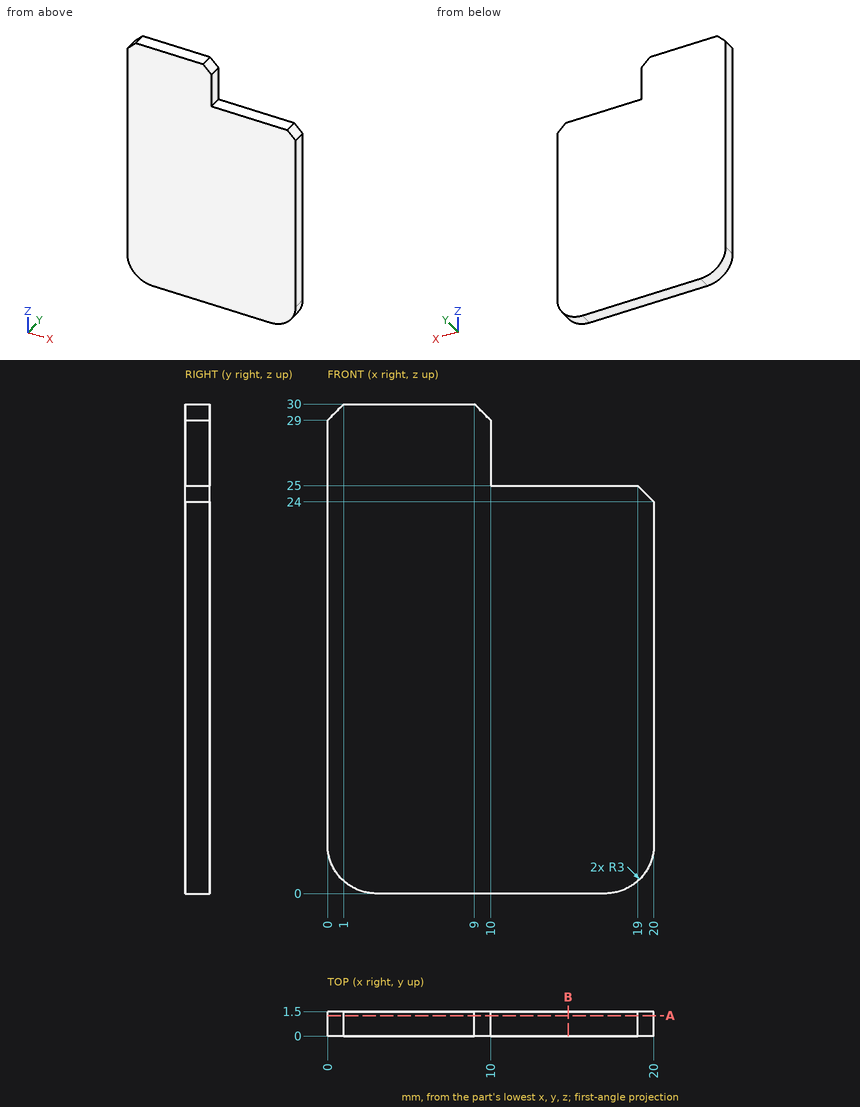
Could you check a few things on this drawing? It's one solid part, dimensions in mm from its lowest x, y, z. Round coordinates to 2 decimals unless told otherwise and drop trailing zeros. Loops run counter-clockwise (first coordinate to the right, second up) from the corner with the lowest first, then second, coordinate; pieces in that order, holes last.
Q1. I want a section at B-B (x = 14.75). Write out the boundary of the cut face in (y, z), and give its area (3 significant figures).
Q2. For P1, Ø0.8, axis at y = 1, z = 26, coming from the +X side, with a flat end and sliding along its axis, tell me the tip position at first contact or that it passes through.
Q3. I want a section at A-A (y = 1.25). Write out the boundary of the cut face in (x, z), and give its area (3 significant figures).
Q4. Please list where these lines run through material, in increasing order: L1, parallel to Z at x = 11.25, y = 0.8; L2, parallel to X at y = 1.3, z = 27.5; L3, parallel to X at y = 0.65, z = 2.25.
Answer below:
1. outline: (0, 0) - (1.5, 0) - (1.5, 25) - (0, 25) - close
1. area: 37.5 mm2
2. P1: stops at x = 10
3. outline: (0, 3) arc R3 ccw to (3, 0) - (17, 0) arc R3 ccw to (20, 3) - (20, 24) - (19, 25) - (10, 25) - (10, 29) - (9, 30) - (1, 30) - (0, 29) - close
3. area: 545 mm2
4. L1: z = 0 to 25
4. L2: x = 0 to 10
4. L3: x = 0.1 to 19.9
